Could you check a few things on this model? Use its own coordinates, in mm. Face numbers are marked on the shaded views. A direction names the side the tool comes from. Round coordinates to 2 decimals unless told otherwise and drop trailing zeros. Loops run counter-clockwise (first coordinate to the right, second up) from the corner with the lowest first, then second, coordinate; pieces in that order, holes last. Notation, with made-up numbers: (-23.5, 3.5) -> (17.5, 3.5) arc R9 cw to (17.5, 13.5) -> close; hole circle Ø4 at (16, -19.75). An arc over 180 degrees is marked (long way). Put each result on its own line as item: value. Start each with the question number.
1. I need wall thicknesses on line 1 (X direction, y = -34.5, z = 4.5); line 2 (Y direction, x = -18.5, z = 2.5); line 3 (X direction, y = -35.5, z = 24.5). Which ranges of each line are inside material? Lowest first, please. Write a range as [from, to].
2. Imagine slicing it at D-D, the plane y = -30. Please give me the cut outline in (x, z).
3. Imagine slicing it at C-C, the plane y = -11.5. Please give me the cut outline in (x, z), and give its area (3 significant figures).
4. Imagine slicing it at B-B, the plane y = -17.5. Please give me the cut outline in (x, z), and give its area (3 significant figures).
5. I'm going to push flat-ended pins straight in: P1, Ø1, axis at x = -10.5, y = -32, coming from the -Z side; P2, Ø1.5, axis at x = 18, y = -4.5, coming from the -Z side; P3, Ø12, axis at y = -24.5, z = 24.5, coming from the -X side; P4, Ø4, axis at y = -34.5, z = 26, coming from the -X side. Where does each tip first touch, or does it pass through?
6. Imagine slicing it at A-A, the plane z = -18. Please give me the cut outline in (x, y).
7. If we mould it in two halves opening along X, with no side actions, what happens to the marked faces 3, 4 and 5? For each: pulls with the +X half, pulls with the -X half, needs draft (parallel to the pull), parting line crosses it, or undercut.
8. Which directions (+Z, -Z, +X, -X, +Y, -Y) give clear straight access to the entire face, cutting with the end or side of a thin tool? Please do the marked faces 1 and 2.
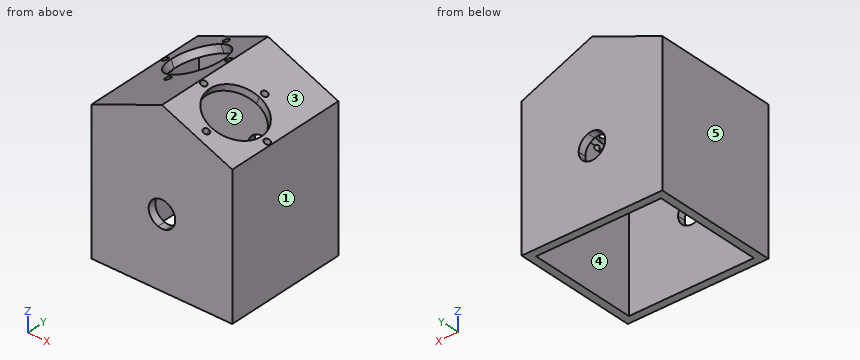
```python
from build123d import *

# Parameters (mm, degrees)
F0_W     = 2.5
F0_H     = 40
F0_H_2   = 2.5
F1_DEPTH = 40
F2_T     = -2.5
F3_DEPTH = 40
F5_R     = 1
F6_DEPTH = 3.5
F4_R     = 1
F7_DEPTH = 3.5


with BuildPart() as f1:
    # F0 (on Front) → F1 (new body)
    with BuildSketch(Plane.XZ):
        Polygon((20, 20), (20, 22.5), (-22.5, 22.5), (-22.5, -22.5), (20, -22.5), (20, -20), (17.5, -20), (17.5, 20), align=None)
        with Locations((-18.75, 0)):
            Rectangle(F0_W, F0_H, mode=Mode.SUBTRACT)
        with Locations((-12.5, 0)):
            Rectangle(F0_W, F0_H, mode=Mode.SUBTRACT)
        with BuildLine():
            Line((1.25, 20), (1.25, 6.6332495807))
            ThreePointArc((1.25, 6.6332495807), (3.2964706517, 5.8903124911), (5, 4.5345892868))
            Line((5, 4.5345892868), (5, 20))
            Line((5, 20), (7.5, 20))
            Line((7.5, 20), (7.5, -20))
            Line((7.5, -20), (5, -20))
            Line((5, -20), (5, -4.5345892868))
            ThreePointArc((5, -4.5345892868), (3.2964706517, -5.8903124911), (1.25, -6.6332495807))
            Line((1.25, -6.6332495807), (1.25, -20))
            Line((1.25, -20), (-1.25, -20))
            Line((-1.25, -20), (-1.25, -6.6332495807))
            ThreePointArc((-1.25, -6.6332495807), (-3.2964706517, -5.8903124911), (-5, -4.5345892868))
            Line((-5, -4.5345892868), (-5, -20))
            Line((-5, -20), (-7.5, -20))
            Line((-7.5, -20), (-7.5, 20))
            Line((-7.5, 20), (-5, 20))
            Line((-5, 20), (-5, 4.5345892868))
            ThreePointArc((-5, 4.5345892868), (-3.2964706517, 5.8903124911), (-1.25, 6.6332495807))
            Line((-1.25, 6.6332495807), (-1.25, 20))
            Line((-1.25, 20), (1.25, 20))
        make_face(mode=Mode.SUBTRACT)
        with Locations((12.5, 0)):
            Rectangle(F0_W, F0_H, mode=Mode.SUBTRACT)
        Polygon((20, 22.5), (22.5, 22.5), (0, 31.8198051534), (-22.5, 22.5), align=None)
        with Locations((-12.5, 0)):
            Rectangle(F0_W, F0_H)
        with Locations((18.75, 0)):
            Rectangle(F0_W, F0_H)
        with Locations((-18.75, 0)):
            Rectangle(F0_W, F0_H)
        with Locations((21.25, 0)):
            Rectangle(F0_W, F0_H)
        with Locations((12.5, 0)):
            Rectangle(F0_W, F0_H)
        with BuildLine():
            Line((5, 20), (5, 4.5345892868))
            ThreePointArc((5, 4.5345892868), (6.2973208589, 2.4302777619), (6.75, 0))
            ThreePointArc((6.75, 0), (6.2973208589, -2.4302777619), (5, -4.5345892868))
            Line((5, -4.5345892868), (5, -20))
            Line((5, -20), (7.5, -20))
            Line((7.5, -20), (7.5, 20))
            Line((7.5, 20), (5, 20))
        make_face()
        with BuildLine():
            ThreePointArc((-5, -4.5345892868), (-6.75, 0), (-5, 4.5345892868))
            Line((-5, 4.5345892868), (-5, 20))
            Line((-5, 20), (-7.5, 20))
            Line((-7.5, 20), (-7.5, -20))
            Line((-7.5, -20), (-5, -20))
            Line((-5, -20), (-5, -4.5345892868))
        make_face()
        with BuildLine():
            ThreePointArc((-1.25, 6.6332495807), (0, 6.75), (1.25, 6.6332495807))
            Line((1.25, 6.6332495807), (1.25, 20))
            Line((1.25, 20), (-1.25, 20))
            Line((-1.25, 20), (-1.25, 6.6332495807))
        make_face()
        with BuildLine():
            Line((1.25, -20), (1.25, -6.6332495807))
            ThreePointArc((1.25, -6.6332495807), (0, -6.75), (-1.25, -6.6332495807))
            Line((-1.25, -6.6332495807), (-1.25, -20))
            Line((-1.25, -20), (1.25, -20))
        make_face()
        with BuildLine():
            ThreePointArc((-1.25, -4.0620192023), (-4.25, 0), (-1.25, 4.0620192023))
            Line((-1.25, 4.0620192023), (-1.25, 6.6332495807))
            ThreePointArc((-1.25, 6.6332495807), (-3.2964706517, 5.8903124911), (-5, 4.5345892868))
            Line((-5, 4.5345892868), (-5, -4.5345892868))
            ThreePointArc((-5, -4.5345892868), (-3.2964706517, -5.8903124911), (-1.25, -6.6332495807))
            Line((-1.25, -6.6332495807), (-1.25, -4.0620192023))
        make_face()
        with BuildLine():
            ThreePointArc((1.25, 4.0620192023), (3.4186985828, 2.5248762346), (4.25, 0))
            ThreePointArc((4.25, 0), (3.4186985828, -2.5248762346), (1.25, -4.0620192023))
            Line((1.25, -4.0620192023), (1.25, -6.6332495807))
            ThreePointArc((1.25, -6.6332495807), (3.2964706517, -5.8903124911), (5, -4.5345892868))
            Line((5, -4.5345892868), (5, 4.5345892868))
            ThreePointArc((5, 4.5345892868), (3.2964706517, 5.8903124911), (1.25, 6.6332495807))
            Line((1.25, 6.6332495807), (1.25, 4.0620192023))
        make_face()
        with BuildLine():
            Line((1.25, -4.0620192023), (1.25, 4.0620192023))
            ThreePointArc((1.25, 4.0620192023), (0, 4.25), (-1.25, 4.0620192023))
            Line((-1.25, 4.0620192023), (-1.25, -4.0620192023))
            ThreePointArc((-1.25, -4.0620192023), (0, -4.25), (1.25, -4.0620192023))
        make_face()
        with BuildLine():
            Line((-1.25, -4.0620192023), (-1.25, 4.0620192023))
            ThreePointArc((-1.25, 4.0620192023), (-4.25, 0), (-1.25, -4.0620192023))
        make_face()
        with BuildLine():
            ThreePointArc((1.25, -4.0620192023), (3.4186985828, -2.5248762346), (4.25, 0))
            ThreePointArc((4.25, 0), (3.4186985828, 2.5248762346), (1.25, 4.0620192023))
            Line((1.25, 4.0620192023), (1.25, -4.0620192023))
        make_face()
        with BuildLine():
            ThreePointArc((6.75, 0), (6.2973208589, 2.4302777619), (5, 4.5345892868))
            Line((5, 4.5345892868), (5, -4.5345892868))
            ThreePointArc((5, -4.5345892868), (6.2973208589, -2.4302777619), (6.75, 0))
        make_face()
        with BuildLine():
            Line((-5, -4.5345892868), (-5, 4.5345892868))
            ThreePointArc((-5, 4.5345892868), (-6.75, 0), (-5, -4.5345892868))
        make_face()
        with BuildLine():
            Line((1.25, -6.6332495807), (1.25, -4.0620192023))
            ThreePointArc((1.25, -4.0620192023), (0, -4.25), (-1.25, -4.0620192023))
            Line((-1.25, -4.0620192023), (-1.25, -6.6332495807))
            ThreePointArc((-1.25, -6.6332495807), (0, -6.75), (1.25, -6.6332495807))
        make_face()
        with BuildLine():
            ThreePointArc((-1.25, 4.0620192023), (0, 4.25), (1.25, 4.0620192023))
            Line((1.25, 4.0620192023), (1.25, 6.6332495807))
            ThreePointArc((1.25, 6.6332495807), (0, 6.75), (-1.25, 6.6332495807))
            Line((-1.25, 6.6332495807), (-1.25, 4.0620192023))
        make_face()
        with Locations((21.25, -21.25)):
            Rectangle(F0_W, F0_H_2)
        with Locations((21.25, 21.25)):
            Rectangle(F0_W, F0_H_2)
    extrude(amount=F1_DEPTH)

    # F2
    f2_openings = [f1.faces().sort_by_distance(p)[0] for p in [
        (0, -20, -22.5),
    ]]
    offset(amount=F2_T, openings=f2_openings)

    # F0 (on Front) → F3 (cut)
    with BuildSketch(Plane.XZ):
        with BuildLine():
            ThreePointArc((1.25, -4.0620192023), (3.4186985828, -2.5248762346), (4.25, 0))
            ThreePointArc((4.25, 0), (3.4186985828, 2.5248762346), (1.25, 4.0620192023))
            Line((1.25, 4.0620192023), (1.25, -4.0620192023))
        make_face()
        with BuildLine():
            Line((1.25, -4.0620192023), (1.25, 4.0620192023))
            ThreePointArc((1.25, 4.0620192023), (0, 4.25), (-1.25, 4.0620192023))
            Line((-1.25, 4.0620192023), (-1.25, -4.0620192023))
            ThreePointArc((-1.25, -4.0620192023), (0, -4.25), (1.25, -4.0620192023))
        make_face()
        with BuildLine():
            Line((-1.25, -4.0620192023), (-1.25, 4.0620192023))
            ThreePointArc((-1.25, 4.0620192023), (-4.25, 0), (-1.25, -4.0620192023))
        make_face()
    extrude(amount=F3_DEPTH, mode=Mode.SUBTRACT)

    # F5 (on face) → F6 (cut)
    with BuildSketch(Plane(origin=(11.25, 0, 27.1599025767), x_dir=(0.9238795325, 0, -0.3826834324), z_dir=(0.3826834324, 0, 0.9238795325))):
        with BuildLine():
            Line((0, -16.5), (0, -25.5))
            Line((0, -25.5), (9, -25.5))
            ThreePointArc((9, -25.5), (6.3639610307, -19.1360389693), (0, -16.5))
        make_face()
        with BuildLine():
            Line((-9, -25.5), (0, -25.5))
            Line((0, -25.5), (0, -16.5))
            ThreePointArc((0, -16.5), (-6.3639610307, -19.1360389693), (-9, -25.5))
        make_face()
        with BuildLine():
            ThreePointArc((-9, -25.5), (-6.3639610307, -31.8639610307), (0, -34.5))
            Line((0, -34.5), (0, -25.5))
            Line((0, -25.5), (-9, -25.5))
        make_face()
        with BuildLine():
            Line((0, -25.5), (0, -34.5))
            ThreePointArc((0, -34.5), (6.3639610307, -31.8639610307), (9, -25.5))
            Line((9, -25.5), (0, -25.5))
        make_face()
        with Locations((-11, -25.5)):
            Circle(F5_R)
        with BuildLine():
            ThreePointArc((1, -14.5), (-0.7071067812, -13.7928932188), (0, -15.5))
            ThreePointArc((0, -15.5), (0.7071067812, -15.2071067812), (1, -14.5))
        make_face()
        with BuildLine():
            ThreePointArc((12, -25.5), (11, -24.5), (10, -25.5))
            ThreePointArc((10, -25.5), (11, -26.5), (12, -25.5))
        make_face()
        with BuildLine():
            Line((0, -36.5), (0, -37.5))
            ThreePointArc((0, -37.5), (0.7071067812, -37.2071067812), (1, -36.5))
            ThreePointArc((1, -36.5), (0.7071067812, -35.7928932188), (0, -35.5))
            Line((0, -35.5), (0, -36.5))
        make_face()
        with BuildLine():
            ThreePointArc((0, -35.5), (-1, -36.5), (0, -37.5))
            Line((0, -37.5), (0, -36.5))
            Line((0, -36.5), (0, -35.5))
        make_face()
    extrude(amount=-F6_DEPTH, mode=Mode.SUBTRACT)

    # F4 (on face) → F7 (cut)
    with BuildSketch(Plane(origin=(-11.25, 0, 27.1599025767), x_dir=(0.9238795325, 0, 0.3826834324), z_dir=(-0.3826834324, 0, 0.9238795325))):
        with BuildLine():
            ThreePointArc((9, -13.5), (6.3639610307, -7.1360389693), (0, -4.5))
            Line((0, -4.5), (0, -13.5))
            Line((0, -13.5), (9, -13.5))
        make_face()
        with BuildLine():
            Line((0, -13.5), (0, -4.5))
            ThreePointArc((0, -4.5), (-6.3639610307, -7.1360389693), (-9, -13.5))
            Line((-9, -13.5), (0, -13.5))
        make_face()
        with BuildLine():
            Line((0, -22.5), (0, -13.5))
            Line((0, -13.5), (-9, -13.5))
            ThreePointArc((-9, -13.5), (-6.3639610307, -19.8639610307), (0, -22.5))
        make_face()
        with BuildLine():
            Line((9, -13.5), (0, -13.5))
            Line((0, -13.5), (0, -22.5))
            ThreePointArc((0, -22.5), (6.3639610307, -19.8639610307), (9, -13.5))
        make_face()
        with BuildLine():
            ThreePointArc((1, -2.5), (0.7071067812, -1.7928932188), (0, -1.5))
            Line((0, -1.5), (0, -2.5))
            Line((0, -2.5), (0, -3.5))
            ThreePointArc((0, -3.5), (0.7071067812, -3.2071067812), (1, -2.5))
        make_face()
        with BuildLine():
            Line((0, -2.5), (0, -1.5))
            ThreePointArc((0, -1.5), (-1, -2.5), (0, -3.5))
            Line((0, -3.5), (0, -2.5))
        make_face()
        with Locations((-11, -13.5)):
            Circle(F4_R)
        with BuildLine():
            ThreePointArc((1, -24.5), (0.7071067812, -23.7928932188), (0, -23.5))
            ThreePointArc((0, -23.5), (-0.7071067812, -25.2071067812), (1, -24.5))
        make_face()
        with BuildLine():
            ThreePointArc((12, -13.5), (11, -12.5), (10, -13.5))
            ThreePointArc((10, -13.5), (11, -14.5), (12, -13.5))
        make_face()
    extrude(amount=-F7_DEPTH, mode=Mode.SUBTRACT)


solid = f1.part
```
Entries:
1. line 1: [-22.5, -20], [20, 22.5]
1. line 2: [-40, -37.5], [-2.5, 0]
1. line 3: [-17.67, -11.14], [11.14, 17.67]
2. outline: (-22.5, -22.5) -> (-20, -22.5) -> (-20, 20.83) -> (0, 29.11) -> (3.09, 27.83) -> (4.05, 30.14) -> (0, 31.82) -> (-22.5, 22.5) -> close; (17.49, 21.87) -> (20, 20.83) -> (20, -22.5) -> (22.5, -22.5) -> (22.5, 22.5) -> (18.45, 24.18) -> close
3. outline: (-22.5, -22.5) -> (-20, -22.5) -> (-20, 20.83) -> (-18.4, 21.49) -> (-19.36, 23.8) -> (-22.5, 22.5) -> close; (-3.14, 30.52) -> (-2.19, 28.21) -> (0, 29.11) -> (20, 20.83) -> (20, -22.5) -> (22.5, -22.5) -> (22.5, 22.5) -> (0, 31.82) -> close
3. area: 292 mm^2
4. outline: (-22.5, -22.5) -> (-20, -22.5) -> (-20, 20.83) -> (-17.74, 21.76) -> (-18.7, 24.07) -> (-22.5, 22.5) -> close; (-3.8, 30.25) -> (-2.84, 27.94) -> (0, 29.11) -> (6.48, 26.43) -> (7.44, 28.74) -> (0, 31.82) -> close; (14.1, 23.27) -> (20, 20.83) -> (20, -22.5) -> (22.5, -22.5) -> (22.5, 22.5) -> (15.06, 25.58) -> close
4. area: 275 mm^2
5. P1: z = 24.56
5. P2: z = 21.35
5. P3: x = -22.5
5. P4: x = -18.88
6. outline: (-22.5, -40) -> (22.5, -40) -> (22.5, 0) -> (-22.5, 0) -> close; hole (-20, -37.5) -> (20, -37.5) -> (20, -2.5) -> (-20, -2.5) -> close
7. face 3: pulls with the +X half
7. face 4: undercut
7. face 5: pulls with the -X half
8. face 1: +Z, -Z, +X, +Y, -Y
8. face 2: -Z
